For this review, take the finished solid that the model builds, in its own axes (mm). A direction names the side the tool comes from. Coordinates: 2 decimals unless noted, no trailing zeros. Write each loop counter-clockwise with the first axis right and the second up, starting at its lowest first coordinate (ties: lowest second). Pieces come first, ordered by that corner, then holes. Notation, with made-up numbers: M 51,-22 L 88,-22 A25 ccw 88,0 Z; hole C -23.5,32 d2. An arc over 180 degrees is marked long. One line per question, with ' | ' between items.
Autodesk Fusion 360 part; units mm, degrees
sketch "Sketch1" plane through (0, 0, 0) normal (0, 0, 1) x (1, 0, 0)
  line L0 (-25.4, 25.4) -> (25.4, 25.4)
  line L1 (25.4, 25.4) -> (25.4, -25.4)
  line L2 (25.4, -25.4) -> (-25.4, -25.4)
  line L3 (-25.4, -25.4) -> (-25.4, 25.4)
  line L4 (0, 25.4) -> (0, -25.4)
  line L5 (-25.4, 0) -> (25.4, 0)
  circle A0 centre (0, 0) radius 3.175
  dimension "d1" = 6.35
  dimension "d2" = 50.8
  dimension "d3" = 50.8
extrude "Extrude1" add sketch "Sketch1" along normal blind 6.35
sketch "Sketch2" plane through (0, 0, 6.35) normal (0, 0, 1) x (-1, 0, 0)
  line L0 (25.4, 25.4) -> (-25.4, 25.4)
  line L1 (-25.4, 25.4) -> (-25.4, -25.4)
  line L2 (-25.4, -25.4) -> (25.4, -25.4)
  line L3 (25.4, -25.4) -> (25.4, 25.4)
  circle A0 centre (0, 0) radius 3.175
  dimension "d6" = 6.35
hole "Hole1" at (0, 0, 6.35) direction (0, 0, -1) diameter 6.35 depth 6.35 tip angle 118
sketch "Sketch3" plane through (0, 0, 6.35) normal (0, 0, 1) x (-1, 0, 0)
  circle A0 centre (0, 0) radius 3.175
  line L0 (25.4, 25.4) -> (-25.4, 25.4)
  line L1 (-25.4, 25.4) -> (-25.4, -25.4)
  line L2 (-25.4, -25.4) -> (25.4, -25.4)
  line L3 (25.4, -25.4) -> (25.4, 25.4)
  line L4 (19.05, -25.4) -> (19.05, 25.4)
  dimension "d10" = 6.35
extrude "Extrude2" add sketch "Sketch3" along normal blind 44.45 contours L0 L2 L3 L4
sketch "Sketch4" plane through (-25.4, 0, 0) normal (-1, 0, 0) x (0, -1, 0)
  line L0 (-25.4, 0) -> (25.4, 0)
  line L1 (25.4, 0) -> (25.4, 50.8)
  line L2 (25.4, 50.8) -> (-25.4, 50.8)
  line L3 (-25.4, 50.8) -> (-25.4, 0)
  circle A0 centre (-12.7, 38.1) radius 2.3812
  circle A1 centre (12.7, 38.1) radius 2.3812
  circle A2 centre (-12.7, 12.7) radius 2.3812
  circle A3 centre (12.7, 12.7) radius 2.3812
  dimension "d13" = 4.7625
  dimension "d16" = 25.4
  dimension "d17" = -25.4
hole "Hole2" at (-25.4, 12.7, 38.1) at (-25.4, -12.7, 38.1) at (-25.4, -12.7, 12.7) at (-25.4, 12.7, 12.7) direction (1, 0, 0) diameter 6.35 depth 6.35 tip angle 118
sketch "Sketch5" plane through (-25.4, 0, 0) normal (-1, 0, 0) x (0, -1, 0)
  circle A0 centre (12.7, 12.7) radius 3.175
  circle A1 centre (-12.7, 38.1) radius 3.175
  circle A2 centre (12.7, 38.1) radius 3.175
  circle A3 centre (-12.7, 12.7) radius 3.175
  line L0 (-25.4, 0) -> (25.4, 0)
  line L1 (25.4, 0) -> (25.4, 50.8)
  line L2 (25.4, 50.8) -> (-25.4, 50.8)
  line L3 (-25.4, 50.8) -> (-25.4, 0)
fillet "Fillet1" radius 1.27 1 edges at (-19.05, 0, 50.8)
fillet "Fillet2" radius 1.905 1 edges at (-19.05, 0, 6.35)
fillet "Fillet3" radius 1.27 1 edges at (25.4, 0, 6.35)
equation "d13 = ( 3 / 16 ) * 1 in"
1. Take a section at B-B on x = 0. State the section outline as (y, z) points (3 decimals).
Computed values:
outline: M -25.4,0 L -3.175,0 L -3.175,6.35 L -25.4,6.35 Z; M 3.175,0 L 25.4,0 L 25.4,6.35 L 3.175,6.35 Z
2. Clearance check with flat-ended pins moving along their axes: P1, Ø12, axis at y = 8, z = 17.5, coming from the +X side; P2, Ø8, axis at x = -2.5, z = 11.5, coming from the +Y side; P3, Ø20.5, axis at x = 3.5, y = 1.5, coming from the +Z side. State where each tip first meets the part, or that it passes through.
Computed values:
P1: stops at x = -19.05 | P2: passes through | P3: stops at z = 6.35
3. Take a section at A-A on y = 0. State the section outline as (x, z) points (3 decimals).
Computed values:
outline: M -25.4,0 L -3.175,0 L -3.175,6.35 L -17.145,6.35 A1.905 cw -19.05,8.255 L -19.05,49.53 A1.27 ccw -20.32,50.8 L -25.4,50.8 Z; M 3.175,0 L 25.4,0 L 25.4,5.08 A1.27 ccw 24.13,6.35 L 3.175,6.35 Z
4. Machinability: for faces 4 (the flat face through (-21, 25.4, 14)), 5 (the flat face through (-19.05, 0, 29)), which of the approach directions +Z, -Z, +X, -X, +Y, -Y give a long, thin tool a straight path to every point of the face, cutting with its end or side? Answer none if there is none.
Computed values:
face 4: +Z, -Z, +X, -X, +Y | face 5: +Z, +X, +Y, -Y
5. Take a section at D-D on y = 12.7. State the section outline as (x, z) points (3 decimals), plus the area to 3 significant figures.
Computed values:
outline: M -25.4,0 L 25.4,0 L 25.4,5.08 A1.27 ccw 24.13,6.35 L -17.145,6.35 A1.905 cw -19.05,8.255 L -19.05,9.525 L -25.4,9.525 Z; M -25.4,15.875 L -19.05,15.875 L -19.05,34.925 L -25.4,34.925 Z; M -25.4,41.275 L -19.05,41.275 L -19.05,49.53 A1.27 ccw -20.32,50.8 L -25.4,50.8 Z | area: 524 mm2
6. For line 1 along Y through (x, z) = (-23.25, 38.1) (3 decimals); line 2 along Z through (x, y) = (-23, -12.7) (3 decimals); line 3 along Z through (x, y) = (-21, 12), list the stretches that pass through material, from the lowest coordinate up.
Computed values:
line 1: y = -25.4 to -15.875, -9.525 to 9.525, 15.875 to 25.4 | line 2: z = 0 to 9.525, 15.875 to 34.925, 41.275 to 50.8 | line 3: z = 0 to 9.6, 15.8 to 35, 41.2 to 50.8
7. Take a section at C-C on z = 12.7. State the section outline as (x, y) points (3 decimals).
Computed values:
outline: M -25.4,-25.4 L -19.05,-25.4 L -19.05,-15.875 L -25.4,-15.875 Z; M -25.4,-9.525 L -19.05,-9.525 L -19.05,9.525 L -25.4,9.525 Z; M -25.4,15.875 L -19.05,15.875 L -19.05,25.4 L -25.4,25.4 Z
8. Draft analysis for pull direction Z (two halves, no side actions). For faces 1 (the cylindrical face through (-22.18, 14.63, 10.18)), 2 (the flat face through (-21, -25.4, 14)), 3 (the cylindrical face through (-18.507, -0.356, 6.923)), state which applies: pulls with the +Z half, pulls with the -Z half, needs draft (parallel to the pull), parting line crosses it, or undercut.
Computed values:
face 1: undercut | face 2: needs draft | face 3: pulls with the +Z half
